Check sheet for the modelled part. Datum: model origin and axes. Units: mm. Face numbers are marked on the shaded views. A direction names the side the tool comes from. Give positions to 0.01 mm unless a question says otherwise; leave off trailing zeros. Write each loop counter-clockwise with the first axis right and the second up, starting at its lowest first coordinate (ties: lowest second). Pieces come first, ordered by that corner, then holes. Notation, with made-up numbers: (27, 82) -> (39, 82) arc R23 cw to (39, 97) -> close; hole circle Ø3 at (-13.75, 1.5). An arc over 180 degrees is marked (long way). Use a Markdown table: item, result. Add a question column.
1. Scan lines: probe 1 along Y at (x, z) = (19, 10.5); probe 2 along Y at (x, z) = (1, -12); probe 3 along Z at (x, y) = (-29, -20.5). Record each from-to range of solid material in increasing order. Write a range as [from, to].
2. Cross-section at C-C (x = 19.5). Enter the section's corners in (y, z), then the cut area to 3 significant figures.
3. Cross-section at A-A (z = -8). Enter the section's corners in (x, y).
4. Gauge pin test, flat ends, axial feed: P1, Ø10, axis at y = -16.5, z = 5, coming from the +X side; P2, Ø2, axis at y = -9, z = -1, coming from the +X side; P3, Ø4.5, axis at y = -9.5, z = -7.5, coming from the +X side; P4, Ø3, axis at y = -8.5, z = -11.5, coming from the -X side. Record the tip position at first contact, or that the pin passes through.
5. Cross-section at D-D (y = -17). Enter the section's corners in (x, z).
6. Set-up check for the marked faces 4 and 5: record each of +Z, -Z, +X, -X, +Y, -Y from which the full face is reachable in a straight line by a thin tool's end or side.
7. Cross-section at B-B (y = -9.25). Enter the section's corners in (x, z), then the cut area to 3 significant figures.
8. Release check for a two-part mould opening along X. For the marked faces 1, 2 and 3 record: released by +X, released by -X, zero draft, split by the parting line, or undercut.
from build123d import *

# Parameters (mm, degrees)
F1_DEPTH  = 12.7
F4_DEPTH  = 25.4
F5_DEPTH  = 25.4
F7_DEPTH  = 12.7
F9_DEPTH  = 25.4
F10_W     = 2.54
F10_H     = 5.5179311894
F11_DEPTH = 25.4


with BuildPart() as f1:
    # F0 (on Top) → F1 (new body)
    with BuildSketch(Plane.XY):
        with BuildLine():
            Line((44.7565504849, 0), (-44.1434495151, 0))
            ThreePointArc((-44.1434495151, 0), (-55.4417593201, -14.7112042456), (-41.7676718473, -27.2447858006))
            Line((-41.7676718473, -27.2447858006), (47.1323281527, -27.2447858006))
            ThreePointArc((47.1323281527, -27.2447858006), (58.4306379576, -12.5335815549), (44.7565504849, 0))
        make_face()
    extrude(amount=F1_DEPTH)

    # F2 (on face) → F4 (join)
    with BuildSketch(Plane(origin=(0, 0, 0), x_dir=(1, 0, 0), z_dir=(0, 0, -1))):
        with BuildLine():
            Line((47.1323281527, 27.2447858006), (-34.4870686531, 27.2447858006))
            Line((-34.4870686531, 27.2447858006), (-34.4870686531, 0))
            Line((-34.4870686531, 0), (44.7565504849, 0))
            ThreePointArc((44.7565504849, 0), (58.4306379576, 12.5335815549), (47.1323281527, 27.2447858006))
        make_face()
    extrude(amount=F4_DEPTH)

    # F5 (add): a face of the model
    f5_faces = [f1.faces().sort_by_distance(p)[0] for p in [
        (-43.7953743511, -13.5694519924, 0),
    ]]
    extrude(f5_faces, amount=F5_DEPTH)

    # F6 (on face) → F7 (cut)
    with BuildSketch(Plane.XY.offset(12.7)):
        Polygon((30.7856556028, -23.4677214175), (31.0655402243, -3.554351395), (-32.4344597757, -3.554351395), (-32.4344597757, -23.4677214175), align=None)
    extrude(amount=-F7_DEPTH, mode=Mode.SUBTRACT)

    # F8 (on face) → F9 (cut)
    with BuildSketch(Plane(origin=(0, 0, -25.4), x_dir=(1, 0, 0), z_dir=(0, 0, -1))):
        Polygon((5.08, 12.5303016976), (0, 12.5303016976), (-5.058103241, 12.5303016976), (-5.058103241, 7.0123705082), (5.08, 7.0123705082), align=None)
    extrude(amount=-F9_DEPTH, mode=Mode.SUBTRACT)

    # F10 (on face) → F11 (cut)
    with BuildSketch(Plane(origin=(0, 0, -25.4), x_dir=(1, 0, 0), z_dir=(0, 0, -1))):
        with Locations((-6.328103241, 9.7713361029)):
            Rectangle(F10_W, F10_H)
        with Locations((6.35, 9.7713361029)):
            Rectangle(F10_W, F10_H)
    extrude(amount=-F11_DEPTH, mode=Mode.SUBTRACT)


solid = f1.part
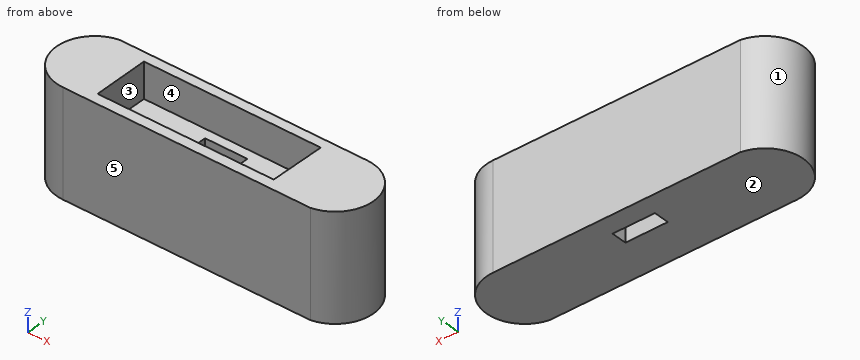
Worked answers:
| question | item | result |
|---|---|---|
| 1 | probe 1 | y = [-27.24, -23.47], [-3.55, 0] |
| 1 | probe 2 | y = [-27.24, -12.53], [-7.01, 0] |
| 1 | probe 3 | z = [-25.4, 0] |
| 2 | outline | (-27.24, -25.4) -> (0, -25.4) -> (0, 12.7) -> (-3.55, 12.7) -> (-3.55, 0) -> (-23.47, 0) -> (-23.47, 12.7) -> (-27.24, 12.7) -> close |
| 2 | area | 785 mm² |
| 3 | outline | (-44.14, 0) arc R13.73 ccw to (-41.77, -27.24) -> (47.13, -27.24) arc R13.73 ccw to (44.76, 0) -> close; hole (-7.6, -12.53) -> (7.62, -12.53) -> (7.62, -7.01) -> (-7.6, -7.01) -> close |
| 4 | P1 | stops at x = 58.48 |
| 4 | P2 | stops at x = 57.97 |
| 4 | P3 | stops at x = 58.34 |
| 4 | P4 | stops at x = -55.03 |
| 5 | outline | (-55.04, -25.4) -> (58.09, -25.4) -> (58.09, 12.7) -> (30.88, 12.7) -> (30.88, 0) -> (-32.43, 0) -> (-32.43, 12.7) -> (-55.04, 12.7) -> close |
| 6 | face 4 | +Z |
| 6 | face 5 | +Z, -Z, +X, -X, -Y |
| 7 | outline | (-54.81, -25.4) -> (-7.6, -25.4) -> (-7.6, 0) -> (-32.43, 0) -> (-32.43, 12.7) -> (-54.81, 12.7) -> close; (7.62, -25.4) -> (57.73, -25.4) -> (57.73, 12.7) -> (30.99, 12.7) -> (30.99, 0) -> (7.62, 0) -> close |
| 7 | area | 3,100 mm² |
| 8 | face 1 | released by -X |
| 8 | face 2 | zero draft |
| 8 | face 3 | undercut |
